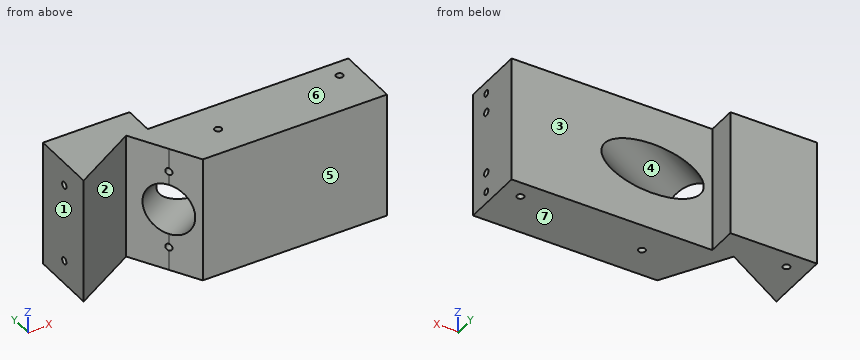
```python
from build123d import *

# Parameters (mm, degrees)
SKETCH1_W                       = 73
SKETCH1_H                       = 32
BOSS_EXTRUDE1_DEPTH             = 16
SKETCH78_W                      = 22
SKETCH78_H                      = 7.5
BOSS_EXTRUDE4_DEPTH             = 32
CUT_EXTRUDE23_DEPTH             = 41
SKETCH14_R                      = 6.5
CUT_EXTRUDE2_DEPTH              = 41
CUT_EXTRUDE2_DEPTH_BACK         = 33
F_2_56_TAPPED_HOLE1_D           = 1.778
F_2_56_TAPPED_HOLE1_DEPTH       = 6.35
F_2_56_TAPPED_HOLE1_TIP         = 0.53416509
F_2_56_TAPPED_HOLE2_D           = 1.778
F_2_56_TAPPED_HOLE2_DEPTH       = 6.35
F_2_56_TAPPED_HOLE2_TIP         = 0.53416509
F_2_56_TAPPED_HOLE3_D           = 1.778
F_2_56_TAPPED_HOLE3_DEPTH       = 6.35
F_2_56_TAPPED_HOLE3_TIP         = 0.53416509
F_2_56_TAPPED_HOLE4_D           = 1.778
F_2_56_TAPPED_HOLE4_DEPTH       = 6.35
F_2_56_TAPPED_HOLE4_TIP         = 0.53416509
F_2_56_TAPPED_HOLE5_D           = 1.778
F_2_56_TAPPED_HOLE5_DEPTH       = 4.76
F_2_56_TAPPED_HOLE5_TIP         = 0.53416509
F_2_56_TAPPED_HOLE7_D           = 1.778
F_2_56_TAPPED_HOLE7_DEPTH       = 15
F_2_56_TAPPED_HOLE7_TIP         = 0.53416509
F_1_16_0_0625_DOWEL_HOLE1_D     = 1.5875
F_1_16_0_0625_DOWEL_HOLE1_DEPTH = 6.5
F_1_16_0_0625_DOWEL_HOLE1_TIP   = 0.476933116


with BuildPart() as part:
    # Sketch1 → Boss-Extrude1 (new body)
    with BuildSketch(Plane(origin=(0, 0, 0), x_dir=(1, 0, 0), z_dir=(0, 1, 0))):
        Rectangle(SKETCH1_W, SKETCH1_H)
    extrude(amount=BOSS_EXTRUDE1_DEPTH)

    # Sketch78 → Boss-Extrude4 (add)
    with BuildSketch(Plane.XY.offset(16)):
        with Locations((-25.5, 19.75)):
            Rectangle(SKETCH78_W, SKETCH78_H)
    extrude(amount=-BOSS_EXTRUDE4_DEPTH)

    # Sketch79 → Cut-Extrude23 (cut)
    with BuildSketch(Plane(origin=(0, 0, -16), x_dir=(-1, 0, 0), z_dir=(0, 0, -1))):
        Polygon((14.495082625, 7.2325), (19.757582625, 16.347417375), (36.5, 6.681178197), (36.5, 0), (10.319396803, 0), align=None)
    extrude(amount=-CUT_EXTRUDE23_DEPTH, mode=Mode.SUBTRACT)

    # Sketch14 → Cut-Extrude2 (cut, two sides)
    with BuildSketch(Plane(origin=(-13.426065962, 5.380908825, -20), x_dir=(0, 0, 1), z_dir=(-0.866025404, -0.5, 0))) as cut_extrude2_sk:
        with Locations((20, 2.138033327)):
            Circle(SKETCH14_R)
    extrude(amount=CUT_EXTRUDE2_DEPTH, mode=Mode.SUBTRACT)
    extrude(cut_extrude2_sk.sketch, amount=-CUT_EXTRUDE2_DEPTH_BACK, mode=Mode.SUBTRACT)

    # #2-56 Tapped Hole1
    with Locations(Plane.ZY.offset(36.5)):
        with Locations((-10, 14.681178197), (10, 14.681178197)):
            Hole(F_2_56_TAPPED_HOLE1_D / 2, depth=F_2_56_TAPPED_HOLE1_DEPTH)
            with Locations((0, 0, -(F_2_56_TAPPED_HOLE1_DEPTH + F_2_56_TAPPED_HOLE1_TIP / 2))):  # 118° drill point
                Cone(0, F_2_56_TAPPED_HOLE1_D / 2, F_2_56_TAPPED_HOLE1_TIP, mode=Mode.SUBTRACT)

    # #2-56 Tapped Hole2
    with Locations(Plane(origin=(0, 0, -16), x_dir=(-1, 0, 0), z_dir=(0, 0, -1))):
        with Locations((-31.5, 11.5), (1.5, 8)):
            Hole(F_2_56_TAPPED_HOLE2_D / 2, depth=F_2_56_TAPPED_HOLE2_DEPTH)
            with Locations((0, 0, -(F_2_56_TAPPED_HOLE2_DEPTH + F_2_56_TAPPED_HOLE2_TIP / 2))):  # 118° drill point
                Cone(0, F_2_56_TAPPED_HOLE2_D / 2, F_2_56_TAPPED_HOLE2_TIP, mode=Mode.SUBTRACT)

    # #2-56 Tapped Hole3
    with Locations(Plane.XY.offset(16)):
        with Locations((-1.5, 8), (31.5, 11.5)):
            Hole(F_2_56_TAPPED_HOLE3_D / 2, depth=F_2_56_TAPPED_HOLE3_DEPTH)
            with Locations((0, 0, -(F_2_56_TAPPED_HOLE3_DEPTH + F_2_56_TAPPED_HOLE3_TIP / 2))):  # 118° drill point
                Cone(0, F_2_56_TAPPED_HOLE3_D / 2, F_2_56_TAPPED_HOLE3_TIP, mode=Mode.SUBTRACT)

    # #2-56 Tapped Hole4
    with Locations(Plane(origin=(-7.739547602, -4.468429892, 0), x_dir=(0, 0, 1), z_dir=(-0.866025404, -0.5, 0))):
        with Locations((-10, 13.511070046), (10, 13.511070046), (0, 13.511070046)):
            Hole(F_2_56_TAPPED_HOLE4_D / 2, depth=F_2_56_TAPPED_HOLE4_DEPTH)
            with Locations((0, 0, -(F_2_56_TAPPED_HOLE4_DEPTH + F_2_56_TAPPED_HOLE4_TIP / 2))):  # 118° drill point
                Cone(0, F_2_56_TAPPED_HOLE4_D / 2, F_2_56_TAPPED_HOLE4_TIP, mode=Mode.SUBTRACT)

    # #2-56 Tapped Hole5
    with Locations(Plane(origin=(0, 0, -16), x_dir=(-1, 0, 0), z_dir=(0, 0, -1))):
        with Locations((31.5, 19)):
            Hole(F_2_56_TAPPED_HOLE5_D / 2, depth=F_2_56_TAPPED_HOLE5_DEPTH)
            with Locations((0, 0, -(F_2_56_TAPPED_HOLE5_DEPTH + F_2_56_TAPPED_HOLE5_TIP / 2))):  # 118° drill point
                Cone(0, F_2_56_TAPPED_HOLE5_D / 2, F_2_56_TAPPED_HOLE5_TIP, mode=Mode.SUBTRACT)

    # #2-56 Tapped Hole7
    with Locations(Plane(origin=(36.5, 0, 0), x_dir=(0, 0, -1), z_dir=(1, 0, 0))):
        with Locations((-8, 5.5), (8, 5.5)):
            Hole(F_2_56_TAPPED_HOLE7_D / 2, depth=F_2_56_TAPPED_HOLE7_DEPTH)
            with Locations((0, 0, -(F_2_56_TAPPED_HOLE7_DEPTH + F_2_56_TAPPED_HOLE7_TIP / 2))):  # 118° drill point
                Cone(0, F_2_56_TAPPED_HOLE7_D / 2, F_2_56_TAPPED_HOLE7_TIP, mode=Mode.SUBTRACT)

    # 1/16 (0.0625) Dowel Hole1
    with Locations(Plane(origin=(36.5, 0, 0), x_dir=(0, 0, -1), z_dir=(1, 0, 0))):
        with Locations((13, 5.5), (-13, 5.5)):
            Hole(F_1_16_0_0625_DOWEL_HOLE1_D / 2, depth=F_1_16_0_0625_DOWEL_HOLE1_DEPTH)
            with Locations((0, 0, -(F_1_16_0_0625_DOWEL_HOLE1_DEPTH + F_1_16_0_0625_DOWEL_HOLE1_TIP / 2))):  # 118° drill point
                Cone(0, F_1_16_0_0625_DOWEL_HOLE1_D / 2, F_1_16_0_0625_DOWEL_HOLE1_TIP, mode=Mode.SUBTRACT)


solid = part.part
```
Build history of the part. All positions in model axes, mm. Face numbers are marked on the shaded views. A direction names the side the tool comes from. Coordinates: 2 decimals unless noted, no trailing zeros. Order: outer loops, then holes, each group sorted by start corner. A loop starts at its lowest first (then second) coordinate and runs counter-clockwise, first axis right, second up.
Item 1: Saw through at A-A on z = 2.5. List the corners of the cut face in (x, y), then the cut area to 3 significant figures.
Filled in:
outline: (-36.5, 6.68) - (-19.76, 16.35) - (-17.5, 12.43) - (-11.31, 16) - (-14.5, 16) - (-14.5, 23.5) - (-36.5, 23.5) - close; (-11.5, 2.04) - (-10.32, 0) - (36.5, 0) - (36.5, 16) - (12.69, 16) - close
area: 853 mm2
Item 2: Drill centre lines: L1, parallel to Z at x = 32, y = 5.5; L2, parallel to Y at x = 31.5, z = 11.75; L3, parallel to Z at x = -31.5, y = 14.5. Where is each one in solid material? Low to high.
Filled in:
L1: z = -16 to -13.79, -12.21 to -8.89, -7.11 to 7.11, 8.89 to 12.21, 13.79 to 16
L2: y = 0 to 10.61, 12.39 to 16
L3: z = -16 to -10.87, -9.13 to 9.13, 10.87 to 16
Item 3: Drop flat-ended pins along their axis: pin 1 Ø1.1 at (x, y) = (-1.5, 8) entering from -Z; pin 2 Ø12 at (x, z) = (14, -1.5) entering from +Y; pin 3 Ø1.6 at (y, z) = (5.5, 8) entering from +X. Give the stop position or say it passes through.
Filled in:
pin 1: stops at z = -9.45
pin 2: stops at y = 16
pin 3: stops at x = 21.45
Item 4: Mould opens along Z. For the marked faces 4, 5, 6 and 7 say: released by +Z, released by -Z, zero draft, split by the parting line, or undercut.
Filled in:
face 4: undercut
face 5: zero draft
face 6: released by +Z
face 7: released by -Z
Item 5: Tool access for the marked faces 1, 2 and 3: list every direction of +Z, -Z, +X, -X, +Y, -Y with a clear straight run to the whole face (end or side of a thin tool).
Filled in:
face 1: +Z, -Z, -X, +Y, -Y
face 2: +Z, -Z, -Y
face 3: +Z, -Z, +X, +Y
Item 6: Saw through at B-B on z = -1.5. List the corners of the cut face in (x, y).
Filled in:
outline: (-36.5, 6.68) - (-19.76, 16.35) - (-17.66, 12.71) - (-11.96, 16) - (-14.5, 16) - (-14.5, 23.5) - (-36.5, 23.5) - close; (-11.33, 1.76) - (-10.32, 0) - (36.5, 0) - (36.5, 16) - (13.34, 16) - close
